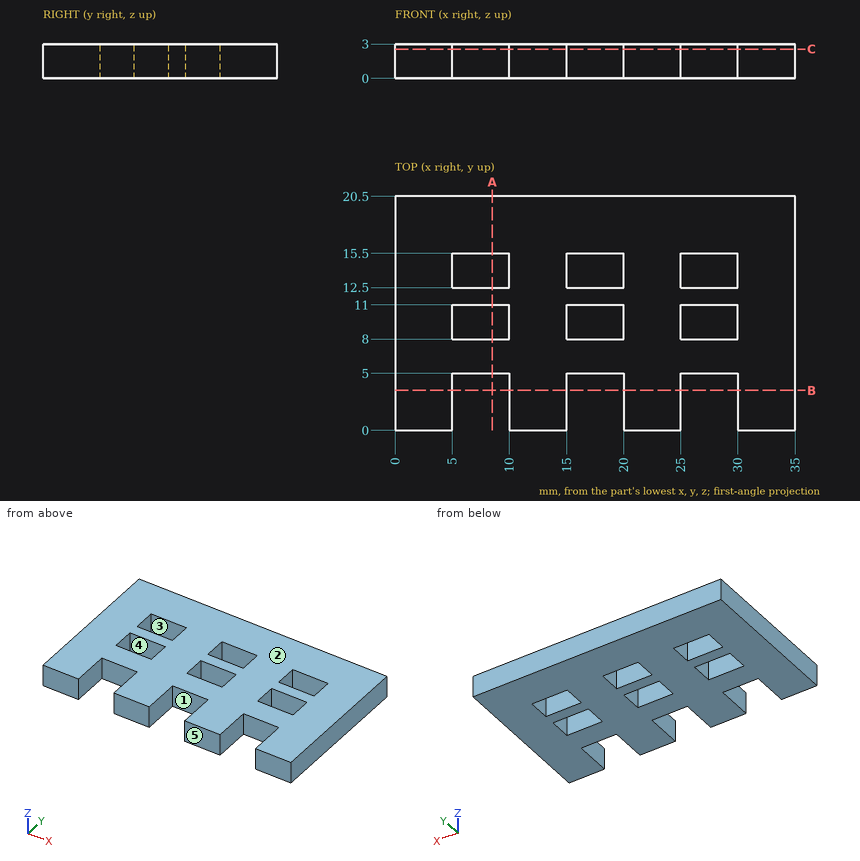
Print and shaded views of the part. All mm, measured from the part's lowest x, y and z. A direction names the side the tool comes from. Round coordinates to 2 decimals unless told otherwise and drop trailing zeros. Write each loop counter-clockwise with the first axis right and the second up, starting at its lowest first coordinate (ties: lowest second). Pieces come first, ordered by that corner, then holes. Notation, with made-up numbers: (69, -7) - (89, -7) arc R25 ccw to (89, 20) - close; hole circle Ø1 at (-28.75, 21.5). An arc over 180 degrees is marked (long way). Write each question's results on one line, items separated by ' | '. Start each with the question number.
Item 1: Mould opens along X. For the marked faces 4 and 5 say: pulls with the +X half, pulls with the -X half, needs draft (parallel to the pull), parting line crosses it, or undercut.
Item 2: Saw through at A-A (x = 8.5). Write the cut outline in (y, z), and give its area (3 significant figures).
Item 3: Saw through at C-C (z = 2.55). State how many separate pieces and enclosed holes the cut face has, and give its area (4 significant figures).
Item 4: Which spindle directions (+Z, -Z, +X, -X, +Y, -Y) get a long thin tool onto all of the face, cutting with end or side? Do the marked faces 1, 2 and 3. Say none if no direction does.
Item 5: Wall check: L1, parallel to Y at x = 27.5, z = 1.35; L2, parallel to X at y = 10.75, z = 0.7. Give the ranges that are in metal, low to high. Write a range as [from, to].
Item 6: Saw through at B-B (y = 3.5). Write the cut outline in (x, z), and give its area (3 significant figures).
Item 7: Drop a flat-ended pin along its axis: P1, Ø0.9, axis at x = 8.5, z = 1.5, coming from the -Y side. Give the stop position or say it passes through.
Results are:
1) face 4: undercut | face 5: needs draft
2) outline: (5, 0) - (8, 0) - (8, 3) - (5, 3) - close; (11, 0) - (12.5, 0) - (12.5, 3) - (11, 3) - close; (15.5, 0) - (20.5, 0) - (20.5, 3) - (15.5, 3) - close | area: 28.5 mm²
3) separate pieces: 1 | enclosed holes: 6 | area: 552.5 mm²
4) face 1: +Z, -Z, -Y | face 2: +Z, +X, -X, +Y, -Y | face 3: +Z, -Z
5) L1: y = [5, 8], [11, 12.5], [15.5, 20.5] | L2: x = [0, 5], [10, 15], [20, 25], [30, 35]
6) outline: (0, 0) - (5, 0) - (5, 3) - (0, 3) - close; (10, 0) - (15, 0) - (15, 3) - (10, 3) - close; (20, 0) - (25, 0) - (25, 3) - (20, 3) - close; (30, 0) - (35, 0) - (35, 3) - (30, 3) - close | area: 60.0 mm²
7) P1: stops at y = 5
